```python
from build123d import *

# Parameters (mm, degrees)
ESBO_O1_W                = 59
ESBO_O1_H                = 41
RESSALTO_EXTRUS_O1_DEPTH = 10.65
ESBO_O2_R                = 11.45
ESBO_O2_R_2              = 8.72
RESSALTO_EXTRUS_O2_DEPTH = 7.9


with BuildPart() as part:
    # Esboço1 → Ressalto-extrusão1 (new, symmetric)
    with BuildSketch(Plane.XY):
        Rectangle(ESBO_O1_W, ESBO_O1_H)
    extrude(amount=RESSALTO_EXTRUS_O1_DEPTH, both=True)

    # Esboço2 → Ressalto-extrusão2 (add)
    with BuildSketch(Plane.XY.offset(10.65)):
        with Locations((10.85, 0)):
            Circle(ESBO_O2_R)
        with Locations((-16.38, 0)):
            Circle(ESBO_O2_R_2)
    extrude(amount=RESSALTO_EXTRUS_O2_DEPTH)


solid = part.part
```
Work out the finished part from the listing and answer in its coordinate system (mm). A direction names the side the tool comes from. Round coordinates to 2 decimals unless told otherwise and drop trailing zeros. Order: outer loops, then holes, each group sorted by start corner. A loop starts at its lowest first (then second) coordinate and runs counter-clockwise, first axis right, second up.
Q1. A tool of negligible diameter and unlimited length cuts with its end or side. For faces 1 (the flat face through (29.5, 0, 0)), 2 (the flat face through (0, 5, 10.65)), from which of +Z, -Z, +X, -X, +Y, -Y can it reach the whole face along a straight path? Write none if from no direction.
Solution:
face 1: +Z, -Z, +X, +Y, -Y
face 2: +Z
Q2. Given pin 1 Ø8 at (x, y) = (-1.5, 16.5) entering from +Z, flat-ended and moving along its own axis, determine where the tip first touches the part or whether it passes through.
Solution:
pin 1: stops at z = 10.65
Q3. The mould has two halves that part along X. Classify faces 3 (the cylindrical face through (8.37, -11.18, 14.54)), 4 (the flat face through (0, -20.5, 0)), 5 (the cylindrical face through (-8.063, 2.619, 14.545)), 6 (the flat face through (-29.5, 0, 0)): pulls with the +X half, pulls with the -X half, needs draft (parallel to the pull), parting line crosses it, or undercut.
Solution:
face 3: undercut
face 4: needs draft
face 5: undercut
face 6: pulls with the -X half
Q4. A cutting plane is placed at C-C, the plane y = 0. Determine the outline of the cut face in (x, z).
Solution:
outline: (-29.5, -10.65) - (29.5, -10.65) - (29.5, 10.65) - (22.3, 10.65) - (22.3, 18.55) - (-0.6, 18.55) - (-0.6, 10.65) - (-7.66, 10.65) - (-7.66, 18.55) - (-25.1, 18.55) - (-25.1, 10.65) - (-29.5, 10.65) - close
Q5. A cutting plane is placed at D-D, the plane x = 10.85. Determine the outline of the cut face in (y, z).
Solution:
outline: (-20.5, -10.65) - (20.5, -10.65) - (20.5, 10.65) - (11.45, 10.65) - (11.45, 18.55) - (-11.45, 18.55) - (-11.45, 10.65) - (-20.5, 10.65) - close
Q6. A cutting plane is placed at A-A, the plane z = 16.5. Determine the outline of the cut face in (x, y).
Solution:
outline: circle Ø17.44 at (-16.38, 0); circle Ø22.9 at (10.85, 0)
Q7. Find the intervals of material crossed by line 1 along Z through (x, y) = (22.5, 13.5); line 2 along X through (y, z) = (-6.5, 17); line 3 along Y through (x, z) = (11.5, 12), in increasing order.
Solution:
line 1: z = -10.65 to 10.65
line 2: x = -22.19 to -10.57, 1.42 to 20.28
line 3: y = -11.43 to 11.43
Q8. A cutting plane is placed at B-B, the plane x = -16.38. Determine the outline of the cut face in (y, z), then the cut area to 3 significant figures.
Solution:
outline: (-20.5, -10.65) - (20.5, -10.65) - (20.5, 10.65) - (8.72, 10.65) - (8.72, 18.55) - (-8.72, 18.55) - (-8.72, 10.65) - (-20.5, 10.65) - close
area: 1,010 mm2
